Source: CAD feature listing. Evaluate the final solid. Frame: model axes, mm. Round coordinates to 2 decimals unless told otherwise and drop trailing zeros. Order: outer loops, then holes, each group sorted by start corner. A loop starts at its lowest first (then second) coordinate and runs counter-clockwise, first axis right, second up. Notation, with made-up numbers: M 31.5,65.25 L 85.5,65.25 A23 ccw 85.5,104.25 Z; hole C 72,-17 d6. An arc over 180 degrees is marked long. Use CSV: the item, a comma, the result in double quotes. Start each with the question number.
```python
from build123d import *

# Parameters (mm, degrees)
SKETCH_1_W          = 65
SKETCH_1_H          = 55
EXTRUDE_1_DEPTH     = 35
CUT_EXTRUDE_1_DEPTH = 34
SKETCH_3_W          = 65
SKETCH_3_H          = 55
EXTRUDE_2_DEPTH     = 1


with BuildPart() as part:
    # Эскиз1 → Бобышка-Вытянуть1 (new body)
    with BuildSketch(Plane(origin=(0, 0, 0), x_dir=(1, 0, 0), z_dir=(0, 1, 0))):
        with Locations((-23.213428901, -3.437024221)):
            Rectangle(SKETCH_1_W, SKETCH_1_H)
    extrude(amount=EXTRUDE_1_DEPTH)

    # Эскиз2 → Вырез-Вытянуть1 (cut)
    with BuildSketch(Plane(origin=(0, 35, 0), x_dir=(1, 0, 0), z_dir=(0, 1, 0))):
        Polygon((-55.213428901, 23.562975779), (-55.213428901, -29.063319013), (-55.213428901, -30.437024221), (8.786571099, -30.437024221), (8.786571099, 23.562975779), align=None)
    extrude(amount=-CUT_EXTRUDE_1_DEPTH, mode=Mode.SUBTRACT)

    # Эскиз3 → Бобышка-Вытянуть2 (add)
    with BuildSketch(Plane(origin=(0, 35, 0), x_dir=(1, 0, 0), z_dir=(0, 1, 0))):
        with Locations((-23.213428901, -3.437024221)):
            Rectangle(SKETCH_3_W, SKETCH_3_H)
    extrude(amount=EXTRUDE_2_DEPTH)


solid = part.part
```
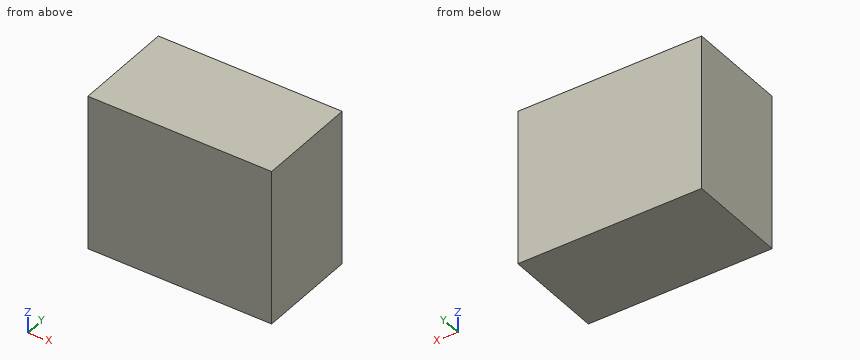
(1) Section B-B on z = -19.5. Return loops of the section in (x, y), plus the area to 3 significant figures.
(2) Section A-A on y = 11. Return loops of the section in (x, z), plus the area to 3 significant figures.
(3) Line query: line 1 along Y through (x, z) = (-20.5, -7); line 2 along X through (y, z) = (14, -6.5); line 3 along Z through (x, y) = (-23, 4.5). Output: solid intervals per line, ascending.
Results below:
1,outline,"M -55.71,0 L 9.29,0 L 9.29,36 L -55.71,36 Z; hole M -55.21,1 L 8.79,1 L 8.79,35 L -55.21,35 Z"
1,area,"164 mm2"
2,outline,"M -55.71,-24.06 L 9.29,-24.06 L 9.29,30.94 L -55.71,30.94 Z; hole M -55.21,-23.56 L 8.79,-23.56 L 8.79,30.44 L -55.21,30.44 Z"
2,area,"119 mm2"
3,line 1,"y = 0 to 1, 35 to 36"
3,line 2,"x = -55.71 to -55.21, 8.79 to 9.29"
3,line 3,"z = -24.06 to -23.56, 30.44 to 30.94"
